Part model, mm, in its own coordinate system. A direction names the side the tool comes from. Coordinates: 2 decimals unless noted, no trailing zeros. Loops run counter-clockwise (first coordinate to the right, second up) from the corner with the lowest first, then second, coordinate; pieces in that order, holes last. Notation, with made-up numbers: M -0.5,25.25 L 20.5,25.25 A16 cw 20.5,32.25 Z; hole C 27,-36 d11. An arc over 180 degrees is marked long. Answer as CSV lines item,"result". Start each with the question number.
from build123d import *

# Parameters (mm, degrees)
F1_DEPTH = 5
F3_D     = 3.3
F3_DEPTH = 13.8
F3_TIP   = 0.9914200214
F4_D     = 5.5
F4_DEPTH = 13.8
F4_TIP   = 1.6523667023
F5_D     = 6.6
F5_DEPTH = 13.8
F5_TIP   = 1.9828400428
F6_R     = 15


with BuildPart() as f1:
    # F0 (on Top) → F1 (new body)
    with BuildSketch(Plane.XY):
        Polygon((140, -125), (200, -125), (200, -87.5), (123.5, -39.6875), (123.5, 39.6875), (200, 87.5), (200, 125), (140, 125), (28, 55), (-28, 55), (-140, 125), (-200, 125), (-200, 87.5), (-123.5, 39.6875), (-123.5, -39.6875), (-200, -87.5), (-200, -125), (-140, -125), (-28, -55), (28, -55), align=None)
    extrude(amount=F1_DEPTH)

    # F3
    with Locations(Plane.XY.offset(5)):
        with Locations((-190, 115), (-190, -115), (190, -115), (190, 115)):
            Hole(F3_D / 2, depth=F3_DEPTH)
            with Locations((0, 0, -(F3_DEPTH + F3_TIP / 2))):  # 118° drill point
                Cone(0, F3_D / 2, F3_TIP, mode=Mode.SUBTRACT)

    # F4
    with Locations(Plane.XY.offset(5)):
        with Locations((50, -30), (50, 30), (10, 20), (10, -20)):
            Hole(F4_D / 2, depth=F4_DEPTH)
            with Locations((0, 0, -(F4_DEPTH + F4_TIP / 2))):  # 118° drill point
                Cone(0, F4_D / 2, F4_TIP, mode=Mode.SUBTRACT)

    # F5
    with Locations(Plane.XY.offset(5)):
        with Locations((-50, 30), (-50, -30)):
            Hole(F5_D / 2, depth=F5_DEPTH)
            with Locations((0, 0, -(F5_DEPTH + F5_TIP / 2))):  # 118° drill point
                Cone(0, F5_D / 2, F5_TIP, mode=Mode.SUBTRACT)

    # F6
    f6_edges = [f1.edges().sort_by_distance(p)[0] for p in [
        (-28, -55, 2.5),
        (28, -55, 2.5),
        (140, -125, 2.5),
        (200, -125, 2.5),
        (200, -87.5, 2.5),
        (123.5, -39.6875, 2.5),
        (123.5, 39.6875, 2.5),
        (200, 87.5, 2.5),
        (200, 125, 2.5),
        (140, 125, 2.5),
        (28, 55, 2.5),
        (-28, 55, 2.5),
        (-140, 125, 2.5),
        (-200, 125, 2.5),
        (-200, 87.5, 2.5),
        (-123.5, 39.6875, 2.5),
        (-123.5, -39.6875, 2.5),
        (-200, -87.5, 2.5),
        (-200, -125, 2.5),
        (-140, -125, 2.5),
    ]]
    fillet(f6_edges, radius=F6_R)


solid = f1.part
Q1. Wall check: L1, parallel to Y at x = 10, z = 3.75; L2, parallel to Y at x = -50, z = 1.7; L3, parallel to X at y = 115, z = 2.15. Give the ranges that are in metal, low to high.
Q2. Flat gauge pins, fed straight in: P1, Ø5.5, axis at x = 190, y = -115, coming from the -Z side; P2, Ø1, axis at x = -127, z = 2, coming from the +Y side; P3, Ø5, axis at x = 50, y = 30, coming from the -Z side; P4, Ø1, axis at x = -76, z = 3.5, coming from the -Y side. Where does each tip first touch, or does it go through?
Q3. Two-plate mould, pull along X, no slides. Class faces 5 (the face through (195.49, -120.72, 2.54)), 6 (the face through (84.733, 90.458, 2.465)), 7 (the face through (-195.72, 120.49, 2.54)): +X half, -X half, draft (parallel to the pull), parting line (faces both ways), or undercut.
Q4. Slice it at C-C, the plane z = 3.15. State how many separate pieces and enclosed holes the cut face has, and give its area (3 significant figures).
Q5. Slice it at D-D, the plane y = -91. Write the cut outline in (x, z), and give its area (3 significant figures).
Q6. Slice it at A-A, the plane y = 78.5. Write the cut outline in (x, z), and give its area (3 significant figures).
Q7. Slice it at B-B, the plane x = -108. Write the cut outline in (y, z).
Q8. Tool access for faces 1 (the face through (-84.733, -90.458, 2.465)), 2 (the face through (162.19, -63.87, 2.46)), 3 (the face through (-162.19, 63.87, 2.46)), 4 (the face through (-83.267, 89.542, 2.465)): list every direction of +Z, -Z, +X, -X, +Y, -Y with a clear straight run to the whole face (end or side of a thin tool).
Solved:
1,L1,"y = -55 to -22.75, -17.25 to 17.25, 22.75 to 55"
1,L2,"y = -68.75 to -33.3, -26.7 to 26.7, 33.3 to 68.75"
1,L3,"x = -199.14 to -191.65, -188.35 to -124, 124 to 188.35, 191.65 to 199.14"
2,P1,"stops at z = 0"
2,P2,"stops at y = 117.19"
2,P3,"passes through"
2,P4,"stops at y = -85.31"
3,face 5,"+X half"
3,face 6,"undercut"
3,face 7,"-X half"
4,separate pieces,"1"
4,enclosed holes,"10"
4,area,"56,600 mm2"
5,outline,"M -199.21,0 L -85.6,0 L -85.6,5 L -199.21,5 Z; M 85.6,0 L 199.21,0 L 199.21,5 L 85.6,5 Z"
5,area,"1,140 mm2"
6,outline,"M -185.6,0 L -65.6,0 L -65.6,5 L -185.6,5 Z; M 65.6,0 L 185.6,0 L 185.6,5 L 65.6,5 Z"
6,area,"1,200 mm2"
7,outline,"M -105,0 L 105,0 L 105,5 L -105,5 Z"
8,face 1,"+Z, -Z, -Y"
8,face 2,"+Z, -Z, +X"
8,face 3,"+Z, -Z, -X"
8,face 4,"+Z, -Z, +Y"
